```python
from build123d import *

# Parameters (mm, degrees)
SKETCH_W     = 40
SKETCH_H     = 32
PAD_DEPTH    = 6
POCKET_DEPTH = 4


with BuildPart() as part:
    # Sketch → Pad (new body)
    with BuildSketch(Plane.XY):
        with Locations((0.861926, -0.003967)):
            Rectangle(SKETCH_W, SKETCH_H)
    extrude(amount=PAD_DEPTH)

    # Sketch001 → Pocket (cut)
    with BuildSketch(Plane.XY.offset(6)):
        Polygon((-6.02844, 15.996033), (-6.02844, -2.599419), (13.97156, -2.599419), (13.97156, 1.400581), (-2.02844, 1.400581), (-2.02844, 15.996033), align=None)
    extrude(amount=-POCKET_DEPTH, mode=Mode.SUBTRACT)


solid = part.part
```
Work out the finished part from the listing and answer in its coordinate system (mm). A direction names the side the tool comes from. Give positions to 0.01 mm unless a question says otherwise; leave off trailing zeros. Loops run counter-clockwise (first coordinate to the right, second up) from the corner with the lowest first, then second, coordinate; pieces in that order, holes last. Notation, with made-up numbers: (68, 27) -> (121, 27) arc R24 cw to (121, 47) -> close; hole circle Ø10 at (63, -40). An arc over 180 degrees is marked (long way). Use CSV: the item, a comma, the result in double quotes.
1. The part is cut by section C-C (z = 3.55). Write down the section's boundary in (x, y).
Found:
outline,"(-19.14, -16) -> (20.86, -16) -> (20.86, 16) -> (-2.03, 16) -> (-2.03, 1.4) -> (13.97, 1.4) -> (13.97, -2.6) -> (-6.03, -2.6) -> (-6.03, 16) -> (-19.14, 16) -> close"
2. The part is cut by section A-A (y = 5.5). Write down the section's boundary in (x, z), then the cut area to 3 significant figures.
Found:
outline,"(-19.14, 0) -> (20.86, 0) -> (20.86, 6) -> (-2.03, 6) -> (-2.03, 2) -> (-6.03, 2) -> (-6.03, 6) -> (-19.14, 6) -> close"
area,"224 mm^2"
3. The part is cut by section B-B (x = -5.5). Write down the section's boundary in (y, z), then the cut area to 3 significant figures.
Found:
outline,"(-16, 0) -> (16, 0) -> (16, 2) -> (-2.6, 2) -> (-2.6, 6) -> (-16, 6) -> close"
area,"118 mm^2"
4. Straight lines are drawn through the part: line 1 (Y direction, x = 2.5, z = 3.3); line 2 (X direction, y = 15.5, z = 4.35); line 3 (Z direction, x = 7, y = -2). For each, find the intervals that lie inside material, in ascending order.
Found:
line 1,"-16 to -2.6, 1.4 to 16"
line 2,"-19.14 to -6.03, -2.03 to 20.86"
line 3,"0 to 2"
5. A tool of negligible diameter and unlimited length cuts with its end or side. For faces 1 (the flat face through (20.862, 0, 3)), 2 (the flat face through (13.972, -1, 4)), 3 (the flat face through (-2.028, 9, 4)), from which of +Z, -Z, +X, -X, +Y, -Y can it reach the whole face along a straight path? Write none if from no direction.
Found:
face 1,"+Z, -Z, +X, +Y, -Y"
face 2,"+Z"
face 3,"+Z, +Y"
6. The mould has two halves that part along Y. Classify faces 4 (the flat face through (1, 0, 0)), 5 (the flat face through (6, 1.401, 4)), 6 (the flat face through (4, -2.599, 4)), 7 (the flat face through (1, -16.004, 3)): +Y half, -Y half, draft (parallel to the pull), parting line (faces both ways), or undercut.
Found:
face 4,"draft"
face 5,"undercut"
face 6,"undercut"
face 7,"-Y half"
7. The part is cut by section D-D (y = -1). Write down the section's boundary in (x, z).
Found:
outline,"(-19.14, 0) -> (20.86, 0) -> (20.86, 6) -> (13.97, 6) -> (13.97, 2) -> (-6.03, 2) -> (-6.03, 6) -> (-19.14, 6) -> close"
